from build123d import *

# Parameters (mm, degrees)
F0_W      = 100
F0_H      = 100
F1_DEPTH  = 140
F3_DEPTH  = 140.001
F5_DEPTH  = 80
F7_W      = 50
F7_H      = 80
F13_DEPTH = 50.00099999
F15_DEPTH = 50.00099999
F16_W     = 30
F16_H     = 59.999
F17_DEPTH = 50


with BuildPart() as f1:
    # F0 (on Top) → F1 (new body)
    with BuildSketch(Plane.XY):
        with Locations((50, 50)):
            Rectangle(F0_W, F0_H)
    extrude(amount=F1_DEPTH)

    # F2 (on face) → F3 (cut, through all)
    with BuildSketch(Plane.XY.offset(140)):
        with BuildLine():
            ThreePointArc((0, 50), (14.6446609407, 85.3553390593), (50, 100))
            Line((50, 100), (0, 100))
            Line((0, 100), (0, 50))
        make_face()
        with BuildLine():
            ThreePointArc((50, 100), (85.3553390593, 85.3553390593), (100, 50))
            Line((100, 50), (100, 100))
            Line((100, 100), (50, 100))
        make_face()
        with BuildLine():
            Line((100, 0), (100, 50))
            ThreePointArc((100, 50), (85.3553390593, 14.6446609407), (50, 0))
            Line((50, 0), (100, 0))
        make_face()
    extrude(amount=-F3_DEPTH, mode=Mode.SUBTRACT)

    # F4 (on face) → F5 (cut)
    with BuildSketch(Plane.XY.offset(140)):
        with BuildLine():
            Line((50, 50), (50, 0))
            ThreePointArc((50, 0), (85.3553390593, 14.6446609407), (100, 50))
            ThreePointArc((100, 50), (50, 100), (0, 50))
            Line((0, 50), (50, 50))
        make_face()
    extrude(amount=-F5_DEPTH, mode=Mode.SUBTRACT)

    # F7 (on face) → F9 section 0
    with BuildSketch(Plane.XZ, mode=Mode.PRIVATE) as f9_s0:
        with Locations((25, 100)):
            Rectangle(F7_W, F7_H)
    loft([f9_s0.sketch, Vertex(0, 30, 140)], mode=Mode.SUBTRACT)

    # F6 (on face) → F10 section 0
    with BuildSketch(Plane.XY.offset(140), mode=Mode.PRIVATE) as f10_s0:
        Polygon((0, 30), (50, 50), (0, 50), align=None)
    loft([f10_s0.sketch, Vertex(50, 50, 60)], mode=Mode.SUBTRACT)

    # F12 (on 3pt) → F13 (cut, through all)
    with BuildSketch(Plane.XZ.offset(-50)):
        Polygon((100, 60), (50.001, 60), (100, 30), align=None)
    extrude(amount=F13_DEPTH, mode=Mode.SUBTRACT)

    # F14 (on 3pt) → F15 (cut, through all)
    with BuildSketch(Plane.XZ.offset(-50)):
        Polygon((100, 0), (100, 29.99), (50.001, 0), align=None)
    extrude(amount=-F15_DEPTH, mode=Mode.SUBTRACT)

    # F16 (on face) → F17 (cut)
    with BuildSketch(Plane(origin=(0, 0, 0), x_dir=(0, -1, 0), z_dir=(-1, 0, 0))):
        with Locations((-15, 29.9995)):
            Rectangle(F16_W, F16_H)
    extrude(amount=-F17_DEPTH, mode=Mode.SUBTRACT)


solid = f1.part
Geometry: final body of the model. Coordinates: model frame, mm. A direction names the side the tool comes from. Round coordinates to 2 decimals unless told otherwise and drop trailing zeros. Loops run counter-clockwise (first coordinate to the right, second up) from the corner with the lowest first, then second, coordinate; pieces in that order, holes last. Notation, with made-up numbers: (-0.75, 13.5) -> (25.25, 13.5) arc R26 ccw to (25.25, 41.5) -> close; hole circle Ø10 at (10, 20.25). An arc over 180 degrees is marked (long way). One line per question, with ' | ' between items. Start each with the question number.
1. Mould query, pull axis X, two halves, no side actions, for faces 1 (the face through (14, 50, 83)), 2 (the face through (14.239, 44.584, 117.218)), 3 (the face through (50, 15, 30)). Classes: pulls with the +X half, pulls with the -X half, needs draft (parallel to the pull), parting line crosses it, or undercut.
2. Set-up query: faces 4 (the face through (25, 30, 30)), 5 (the face through (86, 50, 52)), 6 (the face through (13.539, 8.543, 82.782)). Return all of +Z, -Z, +X, -X, +Y, -Y with unobstructed straight access to the full face (end or side cutting, diameter ignored); none if empty.
3. Contact query for flat-ended pins moving along their axis: pin 1 (12 mm diameter, centred on x = 26.5, z = 112.5, fed in from +Y); pin 2 (8 mm diameter, centred on y = 53.5, z = 41, fed in from +X); pin 3 (5 mm diameter, centred on x = 57, y = 69, fed in from +Z); pin 4 (1 mm diameter, centred on x = 16.5, z = 14, fed in from -Y). Output: stop coordinate, or through.
4. Section C-C on y = 81. Output: boundary loops of the cut face in (x, z), and give its area (3 significant figures).
5. Section D-D on x = 71.5. Output: boundary loops of the cut face in (y, z), and give its area (3 significant figures).
6. Line query: line 1 along X through (y, z) = (25, 124); line 2 along Z through (x, y) = (6.5, 67.5); line 3 along Z through (x, y) = (44.5, 9). Output: solid intervals per line, ascending. Write a range as [from, to].
7. Section A-A on z = 114. Output: boundary loops of the cut face in (x, y), and give its area (3 significant figures).
Returned:
1) face 1: needs draft | face 2: undercut | face 3: pulls with the -X half
2) face 4: -Z, -X, -Y | face 5: +Z, +X, -Y | face 6: +Z, -X, -Y
3) pin 1: stops at y = 43 | pin 2: stops at x = 100 | pin 3: stops at z = 60 | pin 4: stops at y = 30
4) outline: (10.77, 0) -> (50, 0) -> (89.23, 23.53) -> (89.23, 60) -> (10.77, 60) -> close | area: 4,250 mm2
5) outline: (4.86, 0) -> (50, 0) -> (50, 12.9) -> (95.14, 12.9) -> (95.14, 60) -> (50, 60) -> (50, 47.1) -> (4.86, 47.1) -> close | area: 4,250 mm2
6) line 1: x = [0, 50] | line 2: z = [0, 60] | line 3: z = [60, 140]
7) outline: (0, 20.25) -> (16.25, 20.25) -> (50, 0) -> (50, 50) -> (16.25, 36.5) -> (16.25, 50) -> (0, 50) -> close | area: 1,600 mm2
